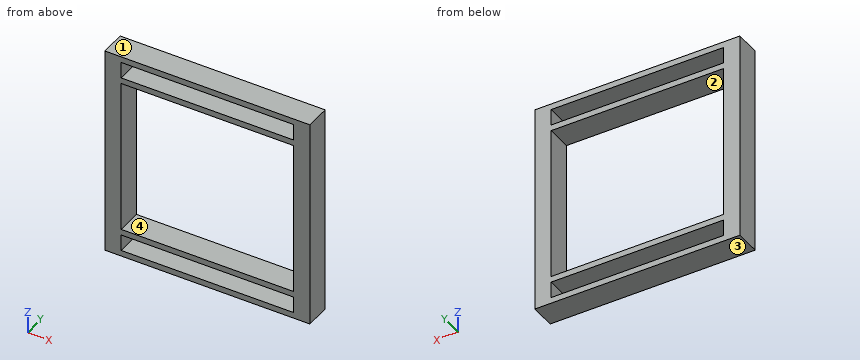
```python
from build123d import *

# Parameters (mm, degrees)
SKETCH1_W           = 701.04
SKETCH1_H           = 721.36
SKETCH1_W_2         = 589.28
SKETCH1_H_2         = 55.88
SKETCH1_H_3         = 528.32
BOSS_EXTRUDE1_DEPTH = 86.36


with BuildPart() as part:
    # Sketch1 → Boss-Extrude1 (new body)
    with BuildSketch(Plane(origin=(0, 0, 0), x_dir=(1, 0, 0), z_dir=(0, 1, 0))):
        Rectangle(SKETCH1_W, SKETCH1_H)
        with Locations((0, 312.42)):
            Rectangle(SKETCH1_W_2, SKETCH1_H_2, mode=Mode.SUBTRACT)
        Rectangle(SKETCH1_W_2, SKETCH1_H_3, mode=Mode.SUBTRACT)
        with Locations((0, -312.42)):
            Rectangle(SKETCH1_W_2, SKETCH1_H_2, mode=Mode.SUBTRACT)
    extrude(amount=BOSS_EXTRUDE1_DEPTH)


solid = part.part
```
Geometry: final body of the model. Coordinates: model frame, mm. Face numbers are marked on the shaded views. A direction names the side the tool comes from. Coordinates: 2 decimals unless noted, no trailing zeros. Order: outer loops, then holes, each group sorted by start corner. A loop starts at its lowest first (then second) coordinate and runs counter-clockwise, first axis right, second up.
Item 1: Draft query along X for the marked faces 3 and 4. Return one class per face: released by +X, released by -X, zero draft, split by the parting line, or undercut.
Answer:
face 3: zero draft
face 4: undercut
Item 2: Section query B-B (z = -155). Output: boundary loops of the cut face in (x, y).
Answer:
outline: (-350.52, 0) - (-294.64, 0) - (-294.64, 86.36) - (-350.52, 86.36) - close; (294.64, 0) - (350.52, 0) - (350.52, 86.36) - (294.64, 86.36) - close
Item 3: Section query C-C (y = 62). Output: boundary loops of the cut face in (x, z), then the cut area to 3 significant figures.
Answer:
outline: (-350.52, -360.68) - (350.52, -360.68) - (350.52, 360.68) - (-350.52, 360.68) - close; hole (-294.64, -340.36) - (294.64, -340.36) - (294.64, -284.48) - (-294.64, -284.48) - close; hole (-294.64, -264.16) - (294.64, -264.16) - (294.64, 264.16) - (-294.64, 264.16) - close; hole (-294.64, 284.48) - (294.64, 284.48) - (294.64, 340.36) - (-294.64, 340.36) - close
area: 129,000 mm2
Item 4: Access query for the marked faces 1 and 2. Directions: +Z, -Z, +X, -X, +Y, -Y. A direction counts if a zero-diameter tool reaches every point of the face in a straight line with its end or side. Return the directions, or none.
Answer:
face 1: +Z, +X, -X, +Y, -Y
face 2: +Y, -Y
Item 5: Material intervals for line 1 along Z through (x, y) = (-185, 59); line 2 along X through (y, z) = (61, 186), sorted ascending.
Answer:
line 1: z = -360.68 to -340.36, -284.48 to -264.16, 264.16 to 284.48, 340.36 to 360.68
line 2: x = -350.52 to -294.64, 294.64 to 350.52
Item 6: Section query A-A (x = 91.5). Output: boundary loops of the cut face in (y, z).
Answer:
outline: (0, -360.68) - (86.36, -360.68) - (86.36, -340.36) - (0, -340.36) - close; (0, -284.48) - (86.36, -284.48) - (86.36, -264.16) - (0, -264.16) - close; (0, 264.16) - (86.36, 264.16) - (86.36, 284.48) - (0, 284.48) - close; (0, 340.36) - (86.36, 340.36) - (86.36, 360.68) - (0, 360.68) - close
